Geometry: final body of the model. Coordinates: model frame, mm. Face numbers are marked on the shaded views. Give positions to 0.01 mm unless a question says otherwise; leave off trailing zeros. Write each loop counter-clockwise with the first axis right and the second up, starting at its lowest first coordinate (ties: lowest second). Pieces come first, ordered by that corner, then holes. Notation, with made-up numbers: M 61.5,-30.5 L 115.5,-30.5 A28 cw 115.5,-11.5 Z; hole C 19,45 d8. An arc over 180 degrees is marked long. One line per question, with ' | ' between items.
from build123d import *

# Parameters (mm, degrees)
SKETCH1_W           = 47
SKETCH1_H           = 55.5
BOSS_EXTRUDE1_DEPTH = 15
CUT_EXTRUDE4_DEPTH  = 54
FILLET1_R           = 7
FILLET2_R           = 7
SKETCH3_W           = 4.401923789
SKETCH3_H           = 6.5
CUT_EXTRUDE5_DEPTH  = 54
SKETCH4_W           = 1
SKETCH4_H           = 1
CUT_EXTRUDE6_DEPTH  = 54
CUT_EXTRUDE7_DEPTH  = 20
CUT_EXTRUDE8_DEPTH  = 5
BOSS_EXTRUDE3_DEPTH = 1.5
CUT_EXTRUDE9_DEPTH  = 57
SKETCH11_W          = 23.5
SKETCH11_H          = 15
CUT_EXTRUDE10_DEPTH = 68.067130548
SKETCH12_W          = 7.286258621
SKETCH12_H          = 11.383570635
BOSS_EXTRUDE4_DEPTH = 10
CUT_EXTRUDE11_DEPTH = 62.343296292


with BuildPart() as part:
    # Sketch1 → Boss-Extrude1 (new body)
    with BuildSketch(Plane(origin=(0, 0, 0), x_dir=(1, 0, 0), z_dir=(0, 1, 0))):
        with Locations((23.5, -27.75)):
            Rectangle(SKETCH1_W, SKETCH1_H)
    extrude(amount=BOSS_EXTRUDE1_DEPTH)

    # Sketch2 → Cut-Extrude4 (cut)
    with BuildSketch(Plane.XY.offset(55.5)):
        with BuildLine():
            ThreePointArc((11.098076211, 15), (8.5, 15.5), (5.901923789, 15))
            Line((5.901923789, 15), (11.098076211, 15))
        make_face()
        with BuildLine():
            Line((11.098076211, 15), (5.901923789, 15))
            ThreePointArc((5.901923789, 15), (4.574858823, 2.70403013), (15.5, 8.5))
            ThreePointArc((15.5, 8.5), (14.29596987, 12.425141177), (11.098076211, 15))
        make_face()
        with BuildLine():
            ThreePointArc((26.098076211, 15), (23.5, 15.5), (20.901923789, 15))
            Line((20.901923789, 15), (26.098076211, 15))
        make_face()
        with BuildLine():
            Line((26.098076211, 15), (20.901923789, 15))
            ThreePointArc((20.901923789, 15), (19.574858823, 2.70403013), (30.5, 8.5))
            ThreePointArc((30.5, 8.5), (29.29596987, 12.425141177), (26.098076211, 15))
        make_face()
        with BuildLine():
            ThreePointArc((45.5, 8.5), (44.29596987, 12.425141177), (41.098076211, 15))
            Line((41.098076211, 15), (35.901923789, 15))
            ThreePointArc((35.901923789, 15), (34.574858823, 2.70403013), (45.5, 8.5))
        make_face()
        with BuildLine():
            Line((35.901923789, 15), (41.098076211, 15))
            ThreePointArc((41.098076211, 15), (38.5, 15.5), (35.901923789, 15))
        make_face()
    extrude(amount=-CUT_EXTRUDE4_DEPTH, mode=Mode.SUBTRACT)

    # Fillet1
    fillet1_edges = [part.edges().sort_by_distance(p)[0] for p in [
        (47, 15, 27.75),
    ]]
    fillet(fillet1_edges, radius=FILLET1_R)

    # Fillet2
    fillet2_edges = [part.edges().sort_by_distance(p)[0] for p in [
        (0, 15, 27.75),
    ]]
    fillet(fillet2_edges, radius=FILLET2_R)

    # Sketch3 → Cut-Extrude5 (cut)
    with BuildSketch(Plane.XY.offset(55.5)):
        with Locations((28.299038106, 11.75)):
            Rectangle(SKETCH3_W, SKETCH3_H)
        with Locations((33.700961895, 11.75)):
            Rectangle(SKETCH3_W, SKETCH3_H)
        with Locations((13.299038106, 11.75)):
            Rectangle(SKETCH3_W, SKETCH3_H)
        with Locations((18.700961895, 11.75)):
            Rectangle(SKETCH3_W, SKETCH3_H)
    extrude(amount=-CUT_EXTRUDE5_DEPTH, mode=Mode.SUBTRACT)

    # Sketch4 → Cut-Extrude6 (cut)
    with BuildSketch(Plane.XY.offset(55.5)):
        with Locations((16, 14.5)):
            Rectangle(SKETCH4_W, SKETCH4_H)
        with Locations((31, 14.5)):
            Rectangle(SKETCH4_W, SKETCH4_H)
    extrude(amount=-CUT_EXTRUDE6_DEPTH, mode=Mode.SUBTRACT)

    # Sketch5 → Cut-Extrude7 (cut)
    with BuildSketch(Plane.ZY.offset(-15.5)):
        Polygon((6.5, 14), (50.5, 14), (40.5, 7), (16.5, 7), align=None)
    extrude(amount=-CUT_EXTRUDE7_DEPTH, mode=Mode.SUBTRACT)

    # Sketch5_2 → Cut-Extrude8 (cut)
    with BuildSketch(Plane.ZY.offset(-15.5)):
        Polygon((6.5, 14), (50.5, 14), (40.5, 7), (16.5, 7), align=None)
    extrude(amount=CUT_EXTRUDE8_DEPTH, mode=Mode.SUBTRACT)

    # Sketch6 → Boss-Extrude3 (add)
    with BuildSketch(Plane.XY.offset(55.5)):
        with BuildLine():
            Line((0, 0), (47, 0))
            Line((47, 0), (47, 8))
            ThreePointArc((47, 8), (44.949747468, 12.949747468), (40, 15))
            Line((40, 15), (7, 15))
            ThreePointArc((7, 15), (2.050252532, 12.949747468), (0, 8))
            Line((0, 8), (0, 0))
        make_face()
    extrude(amount=BOSS_EXTRUDE3_DEPTH)

    # Sketch7 → Cut-Extrude9 (cut)
    with BuildSketch(Plane.XY.offset(57)):
        Polygon((16, 8), (16, 15), (47, 15), (47, 0), (16, 0), align=None)
    extrude(amount=-CUT_EXTRUDE9_DEPTH, mode=Mode.SUBTRACT)

    # Mirror1: part across plane


with BuildPart() as part_1:
    add(part.part)
    add(part.part.mirror(Plane(origin=(16, 8, 0), x_dir=(0, 0, 1), z_dir=(-1, 0, 0))))

    # Sketch11 → Cut-Extrude10 (cut, through all)
    with BuildSketch(Plane.XY.offset(57)):
        with Locations((20.25, 7.5)):
            Rectangle(SKETCH11_W, SKETCH11_H)
    extrude(amount=-CUT_EXTRUDE10_DEPTH, mode=Mode.SUBTRACT)


with BuildPart() as body_2:
    # Sketch12 → Boss-Extrude4 (new body)
    with BuildSketch(Plane.XY.offset(57)):
        with Locations((18.969587134, 9.308214683)):
            Rectangle(SKETCH12_W, SKETCH12_H)
    extrude(amount=BOSS_EXTRUDE4_DEPTH)


with BuildPart() as body_3:
    # Mirror2: mirrored copy
    add(part_1.part.mirror(Plane(origin=(8.5, 15, 0), x_dir=(0, 0, 1), z_dir=(-1, 0, 0))))


with BuildPart() as part_2:
    add(part_1.part)

    # Combine1: union body 3
    add(body_3.part)

    # Sketch13 → Cut-Extrude11 (cut, through all)
    with BuildSketch(Plane(origin=(17, 0, 0), x_dir=(0, 0, -1), z_dir=(1, 0, 0))):
        with BuildLine():
            Line((-38.5, 8), (-18.5, 8))
            ThreePointArc((-18.5, 8), (-15.125235033, 17.548269454), (-6.5, 22.855227978))
            Line((-6.5, 22.855227978), (-18.5, 22.855227978))
            Line((-18.5, 22.855227978), (-38.5, 22.855227978))
            Line((-38.5, 22.855227978), (-50.5, 22.855227978))
            ThreePointArc((-50.5, 22.855227978), (-41.874764967, 17.548269454), (-38.5, 8))
        make_face()
    extrude(amount=-CUT_EXTRUDE11_DEPTH, mode=Mode.SUBTRACT)


solid = part_2.part
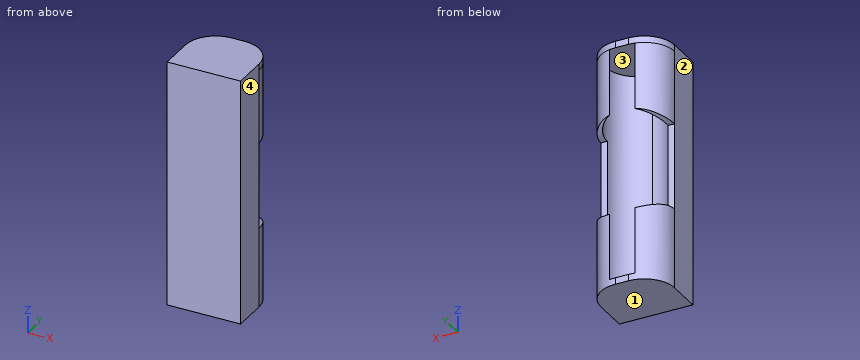
(1) First-contact query: P1, Ø6, axis at x = 6.5, z = 24, coming from the +Y side; P2, Ø0.5, axis at x = 16, z = 25, coming from the +Y side; P3, Ø6.5, axis at x = 10, y = 7.5, coming from the -Z side; P4, Ø4, axis at x = 12, z = 44, coming from the +Y side. Flat tips, straight axial feed; report the tip coordinate or a pass-through.
Working result:
P1: stops at y = 3.6 | P2: stops at y = 8 | P3: stops at z = 0 | P4: stops at y = 14.85
(2) Material intervals for L1, parallel to Z at x = 7.25, y = 11.75; L2, parallel to Y at x = 14.5, z = 47; L3, parallel to X at y = 5.25, z = 17, sorted ascending. Write a range as [from, to].
Working result:
L1: z = [0, 1.5], [55.5, 57] | L2: y = [0, 4.89], [12.11, 13.36] | L3: x = [0, 2.3], [14.7, 17]
(3) Cut plane B-B, the plane z = 25. Return loops of the section in (x, y).
Working result:
outline: M 0,0 L 17,0 L 17,8 L 15.48,8 A7 cw 1.52,8 L 0,8 Z
(4) Cut plane C-C, the plane y = 3.75. Return loops of the section in (x, z).
Working result:
outline: M 0,0 L 17,0 L 17,57 L 0,57 Z; hole M 3.36,1.5 L 13.64,1.5 L 13.64,55.5 L 3.36,55.5 Z
(5) Draft query along X for the marked faces 1, 2, 3 and 4. Return one class per face: released by +X, released by -X, zero draft, split by the parting line, or undercut.
Working result:
face 1: zero draft | face 2: released by -X | face 3: undercut | face 4: released by +X
(6) Cut plane A-A, the plane y = 10.25. Return loops of the section in (x, z).
Working result:
outline: M 0.37,0 L 16.63,0 L 16.63,18.33 L 15.28,18.33 L 15.28,1.5 L 1.72,1.5 L 1.72,18.33 L 0.37,18.33 Z; M 0.37,38.67 L 1.72,38.67 L 1.72,55.5 L 15.28,55.5 L 15.28,38.67 L 16.63,38.67 L 16.63,57 L 0.37,57 Z
(7) Cut plane D-D, the plane x = 3.75. Return loops of the section in (y, z), then the cut area to 3 significant figures.
Working result:
outline: M 0,0 L 14.2,0 L 14.2,17.18 A15.19 ccw 13.64,17.41 L 13.64,1.5 L 3.36,1.5 L 3.36,55.5 L 13.64,55.5 L 13.64,39.59 A15.19 ccw 14.2,39.82 L 14.2,57 L 0,57 Z | area: 242 mm^2
